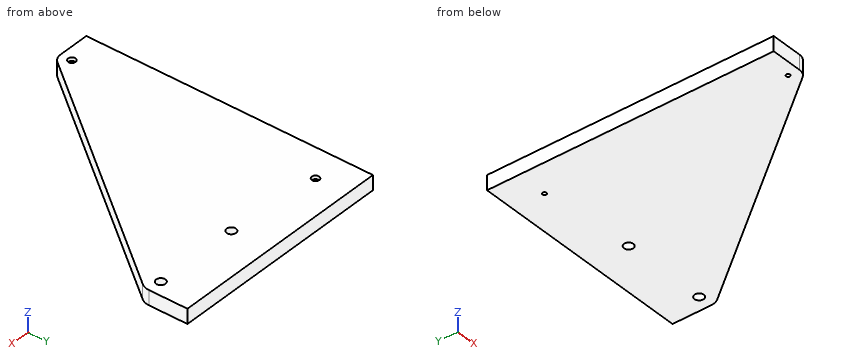
Autodesk Inventor part; units mm, degrees
ref_plane "YZ Plane" through (0, 0, 0) normal (1, 0, 0) x (0, 1, 0)
ref_plane "XZ Plane" through (0, 0, 0) normal (0, 1, 0) x (-1, 0, 0)
ref_plane "XY Plane" through (0, 0, 0) normal (0, 0, 1) x (1, 0, 0)
ref_plane "Work Plane1" through (0, 142.0555, 0) normal (0, 0, 1) x (1, 0, 0)
sketch "Sketch1" plane through (0, 142.0555, 0) normal (0, 0, 1) x (1, 0, 0)
  line L0 (450, -129.5555) -> (450, -142.0555)
  line L1 (0, -129.5555) -> (450, -129.5555)
  line L2 (0, -142.0555) -> (0, -129.5555)
  line L3 (450, -142.0555) -> (0, -142.0555)
  circle A0 centre (109.7339, -163.0555) radius 4.05
  circle A1 centre (184.7339, -163.0555) radius 4.05
  line L4 (92.2339, -147.0555) -> (92.2339, -142.0555)
  arc A2 (97.2339, -152.0555) -> (92.2339, -147.0555) centre (92.2339, -152.0555) ccw
  line L5 (97.2339, -152.0555) -> (97.2339, -163.0555)
  arc A3 (97.2339, -163.0555) -> (122.2339, -163.0555) centre (109.7339, -163.0555) ccw
  line L6 (122.2339, -163.0555) -> (122.2339, -152.0555)
  arc A4 (127.2339, -147.0555) -> (122.2339, -152.0555) centre (127.2339, -152.0555) ccw
  line L7 (127.2339, -147.0555) -> (167.2339, -147.0555)
  arc A5 (172.2339, -152.0555) -> (167.2339, -147.0555) centre (167.2339, -152.0555) ccw
  line L8 (172.2339, -152.0555) -> (172.2339, -163.0555)
  arc A6 (172.2339, -163.0555) -> (197.2339, -163.0555) centre (184.7339, -163.0555) ccw
  line L9 (197.2339, -163.0555) -> (197.2339, -152.0555)
  arc A7 (202.2339, -147.0555) -> (197.2339, -152.0555) centre (202.2339, -152.0555) ccw
  line L10 (202.2339, -142.0555) -> (202.2339, -147.0555)
  line L11 (92.2339, -142.0555) -> (202.2339, -142.0555)
  line L12 (0, -129.5555) -> (0, -379.5555)
  line L13 (0, -379.5555) -> (27.5, -379.5555)
  line L14 (35.3974, -375.6899) -> (194.6057, -170.7235)
  line L15 (197.2339, -163.0555) -> (197.2339, -129.5555)
  line L16 (0, -129.5555) -> (197.2339, -129.5555)
  arc A8 (194.6057, -170.7235) -> (197.2339, -163.0555) centre (184.7339, -163.0555) ccw
  arc A9 (27.5, -379.5555) -> (35.3974, -375.6899) centre (27.5, -369.5555) ccw
  dimension "d2" = 250
  dimension "d5" = 20
  dimension "d6" = 27.5
extrude "Extrusion1" add sketch "Sketch1" along normal blind 12.7508 contours L15 L3 L2 L1 | L15 L9 A6 L8 A5 L7 A4 L6 A3 L5 A2 L4 L3 | L3 L4 A2 L5 A3 L6 A4 L7 A5 L8 A6 L14 A9 L13 L12
sketch "Sketch2" plane through (0, 142.0555, 0) normal (0, 0, -1) x (-1, 0, 0)
  circle A0 centre (-27.5, -369.5555) radius 1.55
  circle A1 centre (-27.5, -157.0555) radius 1.55
  point P0 (0, -142.0555)
extrude "Extrusion2" cut sketch "Sketch2" against normal through all
sketch "Sketch3" plane through (0, 142.0555, 12.7508) normal (0, 0, 1) x (1, 0, 0)
  circle A0 centre (27.5, -157.0555) radius 1.55
  arc A1 (27.5, -379.5555) -> (35.3974, -375.6899) centre (27.5, -369.5555) ccw
  point P0 (0, -142.0555)
hole "Hole1" at (27.5, -15, 12.7508) at (27.5, -227.5, 12.7508) direction (0, 0, -1) diameter 3.4036 end through all counterbore diameter 6.5024 counterbore depth 2.9972
properties part number "side support"
Geometry check sheet. Reference: the model listing, model coordinates, mm. Give positions to 0.01 mm unless a question says otherwise; leave off trailing zeros. Order: outer loops, then holes, each group sorted by start corner. A loop starts at its lowest first (then second) coordinate and runs counter-clockwise, first axis right, second up.
1) Gauge pin test, flat ends, axial feed: pin 1 (4.5 mm diameter, centred on x = 27.5, y = -227.5, fed in from +Z); pin 2 (3 mm diameter, centred on x = 34, z = 3.5, fed in from -Y); pin 3 (4 mm diameter, centred on y = -60, z = 4, fed in from +X). Record the tip position at first contact, or that the pin passes through.
Results are:
pin 1: stops at z = 9.75
pin 2: stops at y = -236.16
pin 3: stops at x = 171.82
2) Cross-section at C-C (y = -133). Record the boundary of the cut face in (x, z).
Results are:
outline: (0, 0) - (113.57, 0) - (113.57, 12.75) - (0, 12.75) - close
3) Cross-section at A-A (z = 2). Record the boundary of the cut face in (x, y).
Results are:
outline: (0, -237.5) - (27.5, -237.5) arc R10 ccw to (35.4, -233.63) - (194.61, -28.67) arc R12.5 ccw to (197.23, -21) - (197.23, 12.5) - (0, 12.5) - close; hole circle Ø3.4 at (27.5, -227.5); hole circle Ø3.4 at (27.5, -15); hole circle Ø8.1 at (109.73, -21); hole circle Ø8.1 at (184.73, -21)
4) Cross-section at B-B (x = 59.5). Record the boundary of the cut face in (y, z), then the cut area to 3 significant figures.
Results are:
outline: (-202.6, 0) - (12.5, 0) - (12.5, 12.75) - (-202.6, 12.75) - close
area: 2,740 mm2
5) Material ranges on probe 1 along Y at (x, z) = (27.5, 5.5); probe 2 along Y at (x, z) = (27.5, 10.5); probe 3 along X at (y, z) = (-227.5, 10.4), recorded low to high.
Results are:
probe 1: y = -237.5 to -229.2, -225.8 to -16.7, -13.3 to 12.5
probe 2: y = -237.5 to -230.75, -224.25 to -18.25, -11.75 to 12.5
probe 3: x = 0 to 24.25, 30.75 to 40.16
